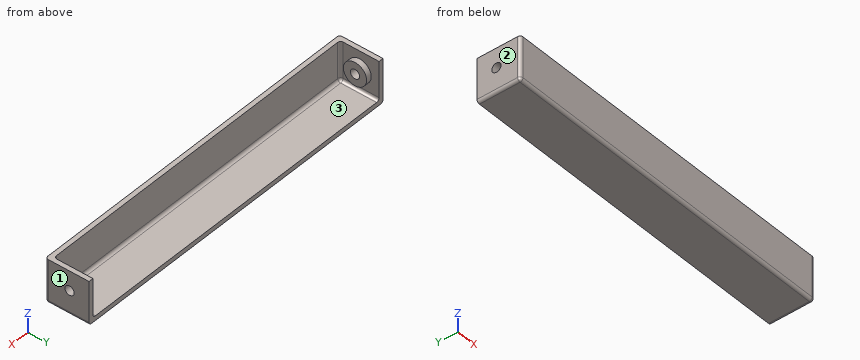
from build123d import *

# Parameters (mm, degrees)
SKETCH_1_W             = 120
SKETCH_1_H             = 15
SM_BASE_FLANGE_1_DEPTH = 1.6
EXTRUDE_1_OUTLINE_W    = 116.8
EXTRUDE_1_OUTLINE_H    = 1.6
EXTRUDE_1_DEPTH        = 13.4
SKETCH_37_5_W          = 1.6
SKETCH_37_5_H          = 15
EXTRUDE_2_DEPTH        = 13.4
SKETCH_45_R            = 4
EXTRUDE_4_DEPTH        = 1.9
SKETCH_46_R            = 1.6
CUT_EXTRUDE_2_DEPTH    = 119.223559412
FILLET_3_R             = 1
FILLET_4_R             = 1


# Read off the part's stored shape, not the designer's step: 拉伸-薄壁1
# Sheet-metal steps are written as plain solids
with BuildPart() as part:
    # Sketch 1 → 基体-法兰1 (new body)
    with BuildSketch(Plane.XY):
        with Locations((0, 7.5)):
            Rectangle(SKETCH_1_W, SKETCH_1_H)
    extrude(amount=-SM_BASE_FLANGE_1_DEPTH)

    # 拉伸-薄壁1 outline → 拉伸-薄壁1 (add)
    with BuildSketch(Plane.XY):
        with Locations((0, 0.8)):
            Rectangle(EXTRUDE_1_OUTLINE_W, EXTRUDE_1_OUTLINE_H)
    extrude(amount=EXTRUDE_1_DEPTH)

    # 草图37<5> → 凸台-拉伸2 (add)
    with BuildSketch(Plane.XY):
        with Locations((-59.2, 7.5)):
            Rectangle(SKETCH_37_5_W, SKETCH_37_5_H)
        with Locations((59.2, 7.5)):
            Rectangle(SKETCH_37_5_W, SKETCH_37_5_H)
    extrude(amount=EXTRUDE_2_DEPTH)

    # 草图45 → 凸台-拉伸4 (add)
    with BuildSketch(Plane.ZY.offset(-58.4)):
        with Locations(Location((6.7, 8.3, 0), (0, 0, 90))):
            Circle(SKETCH_45_R)
    extrude_4 = extrude(amount=EXTRUDE_4_DEPTH)

    # 镜向1: 凸台-拉伸4 across plane
    add(extrude_4.mirror(Plane(origin=(0, 0, 0), x_dir=(0, 0, 1), z_dir=(1, 0, 0))))

    # 草图46 → 切除-拉伸2 (cut, through all)
    with BuildSketch(Plane.ZY.offset(-56.5)):
        with Locations(Location((6.7, 8.3, 0), (0, 0, 270))):
            Circle(SKETCH_46_R)
    cut_extrude_2 = extrude(amount=-CUT_EXTRUDE_2_DEPTH, mode=Mode.SUBTRACT)

    # 镜向2: 切除-拉伸2 across plane
    add(cut_extrude_2.mirror(Plane(origin=(0, 0, 0), x_dir=(0, 0, 1), z_dir=(1, 0, 0))), mode=Mode.SUBTRACT)

    # 圆角3
    fillet_3_edges = [part.edges().sort_by_distance(p)[0] for p in [
        (60, 7.5, -1.6),
        (0, 1.6, 0),
        (58.4, 8.3, 0),
        (-60, 7.5, -1.6),
        (-58.4, 8.3, 0),
        (0, 0, -1.6),
        (60, 0, 5.9),
        (-60, 0, 5.9),
    ]]
    fillet(fillet_3_edges, radius=FILLET_3_R)

    # 圆角4
    # the kernel refuses this fillet: 1 mm, written as the material it adds along each edge
    with BuildSketch(Plane(origin=(-57.4, 2.6, 1), x_dir=(0, -1, 0), z_dir=(-1, 0, 0))) as fillet_4_piece_1_section:
        Polygon((0, 0), (FILLET_4_R, 0), (FILLET_4_R, -FILLET_4_R), (0, -FILLET_4_R), align=None)
    fillet_4_piece_1 = extrude(amount=FILLET_4_R, mode=Mode.PRIVATE)
    fillet_4_piece_1 = fillet_4_piece_1 - Plane(origin=(-57.4, 2.6, 1), x_dir=(0, 0.7071067811865475, 0.7071067811865475), z_dir=(-1, 0, 0)) * Sphere(FILLET_4_R, mode=Mode.PRIVATE)
    add(fillet_4_piece_1)
    with BuildSketch(Plane(origin=(57.4, 2.6, 1), x_dir=(0, -1, 0), z_dir=(1, 0, 0))) as fillet_4_piece_2_section:
        Polygon((0, 0), (FILLET_4_R, 0), (FILLET_4_R, FILLET_4_R), (0, FILLET_4_R), align=None)
    fillet_4_piece_2 = extrude(amount=FILLET_4_R, mode=Mode.PRIVATE)
    fillet_4_piece_2 = fillet_4_piece_2 - Plane(origin=(57.4, 2.6, 1), x_dir=(0, 0.7071067811865475, 0.7071067811865475), z_dir=(1, 0, 0)) * Sphere(FILLET_4_R, mode=Mode.PRIVATE)
    add(fillet_4_piece_2)
    with BuildSketch(Plane(origin=(58.4, 1.6, 1), x_dir=(0, 1, 0), z_dir=(0, 0, 1))) as fillet_4_piece_3:
        with BuildLine():
            CenterArc((FILLET_4_R, FILLET_4_R), FILLET_4_R, 180, 90)
            Line((0, FILLET_4_R), (0, 0))
            Line((0, 0), (FILLET_4_R, 0))
        make_face()
    extrude(amount=12.4)
    with BuildSketch(Plane(origin=(-58.4, 1.6, 1), x_dir=(0, 1, 0), z_dir=(0, 0, 1))) as fillet_4_piece_4:
        with BuildLine():
            CenterArc((FILLET_4_R, -FILLET_4_R), FILLET_4_R, 90, 90)
            Line((0, -FILLET_4_R), (0, 0))
            Line((0, 0), (FILLET_4_R, 0))
        make_face()
    extrude(amount=12.4)


solid = part.part
Could you check a few things on this model? Use its own coordinates, in mm. Face numbers are marked on the shaded views. Round coordinates to 2 decimals unless told otherwise and drop trailing zeros. Order: outer loops, then holes, each group sorted by start corner. A loop starts at its lowest first (then second) coordinate and runs counter-clockwise, first axis right, second up.
(1) If we mould it in two halves opening along X, with no side actions, what happens to the marked faces 1, 2 and 3? For each: released by +X, released by -X, zero draft, split by the parting line, or undercut.
Response values:
face 1: released by +X
face 2: released by -X
face 3: undercut
(2) I'm going to push flat-ended pins straight in: pin 1 (3 mm diameter, centred on y = 8.3, z = 6.7, fed in from +X); pin 2 (3.5 mm diameter, centred on x = -11, z = 10, fed in from +Y); pin 3 (1.5 mm diameter, centred on x = -42, y = 9, fed in from +Z). Where does each tip first touch, or does it pass through?
Response values:
pin 1: passes through
pin 2: stops at y = 1.6
pin 3: stops at z = 0
(3) Imagine slicing it at A-A (z = 6.7). Write out the boundary of the cut face in (x, y), plus the area to 3 significant figures.
Response values:
outline: (-60, 1) arc R1 ccw to (-59, 0) - (59, 0) arc R1 ccw to (60, 1) - (60, 6.7) - (56.5, 6.7) - (56.5, 4.3) - (58.4, 4.3) - (58.4, 2.6) arc R1 cw to (57.4, 1.6) - (-57.4, 1.6) arc R1 cw to (-58.4, 2.6) - (-58.4, 4.3) - (-56.5, 4.3) - (-56.5, 6.7) - (-60, 6.7) - close; (-60, 9.9) - (-56.5, 9.9) - (-56.5, 12.3) - (-58.4, 12.3) - (-58.4, 15) - (-60, 15) - close; (56.5, 9.9) - (60, 9.9) - (60, 15) - (58.4, 15) - (58.4, 12.3) - (56.5, 12.3) - close
area: 243 mm2
(4) Imagine slicing it at B-B (y = 8.3). Write out the boundary of the cut face in (x, z), plus the area to 3 significant figures.
Response values:
outline: (-60, -0.6) arc R1 ccw to (-59, -1.6) - (59, -1.6) arc R1 ccw to (60, -0.6) - (60, 5.1) - (56.5, 5.1) - (56.5, 2.7) - (58.4, 2.7) - (58.4, 1) arc R1 cw to (57.4, 0) - (-57.4, 0) arc R1 cw to (-58.4, 1) - (-58.4, 2.7) - (-56.5, 2.7) - (-56.5, 5.1) - (-60, 5.1) - close; (-60, 8.3) - (-56.5, 8.3) - (-56.5, 10.7) - (-58.4, 10.7) - (-58.4, 13.4) - (-60, 13.4) - close; (56.5, 8.3) - (60, 8.3) - (60, 13.4) - (58.4, 13.4) - (58.4, 10.7) - (56.5, 10.7) - close
area: 243 mm2
(5) Imagine slicing it at C-C (x = 43.5). Write out the boundary of the cut face in (y, z), plus the area to 3 significant figures.
Response values:
outline: (0, -0.6) arc R1 ccw to (1, -1.6) - (15, -1.6) - (15, 0) - (2.6, 0) arc R1 cw to (1.6, 1) - (1.6, 13.4) - (0, 13.4) - close
area: 45.4 mm2
(6) Please list where these lines run through material, in increasing order: line 1 along X through (y, z) = (8.75, 3.5); line 2 along Y through (x, z) = (-59.1, 6.7); line 3 along Z through (x, y) = (-58.25, 8.3).
Response values:
line 1: x = -60 to -56.5, 56.5 to 60
line 2: y = 0.01 to 6.7, 9.9 to 15
line 3: z = -1.6 to 0.47, 2.7 to 5.1, 8.3 to 10.7
